Geometry: final body of the model. Coordinates: model frame, mm. A direction names the side the tool comes from. Coordinates: 2 decimals unless noted, no trailing zeros. Write each loop counter-clockwise with the first axis right and the second up, starting at its lowest first coordinate (ties: lowest second). Pieces come first, ordered by that corner, then holes. Notation, with made-up numbers: (77.5, -0.5) -> (130.5, -0.5) arc R26 cw to (130.5, 35.5) -> close; hole circle Ø10 at (54.5, -32). An arc over 180 degrees is marked (long way). One line per item, written item: value.
```python
from build123d import *

# Parameters (mm, degrees)
F0_R     = 26
F0_R_2   = 7
F1_DEPTH = 3
F2_DEPTH = 15
F3_SIZE2 = 1.819851
F3_SIZE  = 5
F4_SIZE2 = 1.819851
F4_SIZE  = 5


with BuildPart() as f1:
    # F0 (on Top) → F1 (new body)
    with BuildSketch(Plane.XY):
        Circle(F0_R)
        with BuildLine():
            ThreePointArc((3, 22.803509), (17.291616, 15.165751), (23, 0))
            ThreePointArc((23, 0), (22.557855, -4.488117), (21.248418, -8.803678))
            ThreePointArc((21.248418, -8.803678), (19.918584, -11.5), (18.248418, -13.99983))
            ThreePointArc((18.248418, -13.99983), (0, -23), (-18.248418, -13.99983))
            ThreePointArc((-18.248418, -13.99983), (-19.918584, -11.5), (-21.248418, -8.803678))
            ThreePointArc((-21.248418, -8.803678), (-19.918584, 11.5), (-3, 22.803509))
            ThreePointArc((-3, 22.803509), (0, 23), (3, 22.803509))
        make_face(mode=Mode.SUBTRACT)
        with BuildLine():
            Line((-9.761356, -2.17162), (-21.248418, -8.803678))
            ThreePointArc((-21.248418, -8.803678), (-19.918584, -11.5), (-18.248418, -13.99983))
            Line((-18.248418, -13.99983), (-6.761356, -7.367772))
            ThreePointArc((-6.761356, -7.367772), (-8.660254, -5), (-9.761356, -2.17162))
        make_face()
        with BuildLine():
            ThreePointArc((10, 0), (8.062258, 5.91608), (3, 9.539392))
            ThreePointArc((3, 9.539392), (0, 10), (-3, 9.539392))
            ThreePointArc((-3, 9.539392), (-8.660254, 5), (-9.761356, -2.17162))
            ThreePointArc((-9.761356, -2.17162), (-8.660254, -5), (-6.761356, -7.367772))
            ThreePointArc((-6.761356, -7.367772), (0, -10), (6.761356, -7.367772))
            ThreePointArc((6.761356, -7.367772), (8.660254, -5), (9.761356, -2.17162))
            ThreePointArc((9.761356, -2.17162), (9.94016, -1.092347), (10, 0))
        make_face()
        Circle(F0_R_2, mode=Mode.SUBTRACT)
        with BuildLine():
            Line((3, 9.539392), (3, 22.803509))
            ThreePointArc((3, 22.803509), (0, 23), (-3, 22.803509))
            Line((-3, 22.803509), (-3, 9.539392))
            ThreePointArc((-3, 9.539392), (0, 10), (3, 9.539392))
        make_face()
        with BuildLine():
            ThreePointArc((18.248418, -13.99983), (19.918584, -11.5), (21.248418, -8.803678))
            Line((21.248418, -8.803678), (9.761356, -2.17162))
            ThreePointArc((9.761356, -2.17162), (8.660254, -5), (6.761356, -7.367772))
            Line((6.761356, -7.367772), (18.248418, -13.99983))
        make_face()
    extrude(amount=F1_DEPTH)

    # F0 (on Top) → F2 (join)
    with BuildSketch(Plane.XY):
        Circle(F0_R)
        with BuildLine():
            ThreePointArc((3, 22.803509), (17.291616, 15.165751), (23, 0))
            ThreePointArc((23, 0), (22.557855, -4.488117), (21.248418, -8.803678))
            ThreePointArc((21.248418, -8.803678), (19.918584, -11.5), (18.248418, -13.99983))
            ThreePointArc((18.248418, -13.99983), (0, -23), (-18.248418, -13.99983))
            ThreePointArc((-18.248418, -13.99983), (-19.918584, -11.5), (-21.248418, -8.803678))
            ThreePointArc((-21.248418, -8.803678), (-19.918584, 11.5), (-3, 22.803509))
            ThreePointArc((-3, 22.803509), (0, 23), (3, 22.803509))
        make_face(mode=Mode.SUBTRACT)
        with BuildLine():
            ThreePointArc((10, 0), (8.062258, 5.91608), (3, 9.539392))
            ThreePointArc((3, 9.539392), (0, 10), (-3, 9.539392))
            ThreePointArc((-3, 9.539392), (-8.660254, 5), (-9.761356, -2.17162))
            ThreePointArc((-9.761356, -2.17162), (-8.660254, -5), (-6.761356, -7.367772))
            ThreePointArc((-6.761356, -7.367772), (0, -10), (6.761356, -7.367772))
            ThreePointArc((6.761356, -7.367772), (8.660254, -5), (9.761356, -2.17162))
            ThreePointArc((9.761356, -2.17162), (9.94016, -1.092347), (10, 0))
        make_face()
        Circle(F0_R_2, mode=Mode.SUBTRACT)
    extrude(amount=-F2_DEPTH)

    # F3
    f3_edges = [f1.edges().sort_by_distance(p)[0] for p in [
        (-26, 0, -15),
    ]]
    chamfer(f3_edges, length=F3_SIZE, length2=F3_SIZE2)

    # F4
    f4_edges = [f1.edges().sort_by_distance(p)[0] for p in [
        (-7, 0, -15),
    ]]
    chamfer(f4_edges, length=F4_SIZE, length2=F4_SIZE2)


solid = f1.part
```
(1) Reachability of faces 3 (the flat face through (3, 16, 1)), 4 (the flat face through (0, 16, 0)), 5 (the flat face through (0, -9, -15)) from +Z, -Z, +X, -X, +Y, -Y: full face, straight path, thin tool, end or side. Return the list, or none.
Responses:
face 3: +Z, -Z
face 4: -Z
face 5: -Z, +X, -X, +Y, -Y
(2) Pull-direction query (Y, two-part tool) for faces 1 (the flat face through (0, -8, 3)), 2 (the flat face through (-12.585, -10.73, 1.479)); classes: released by +Y, released by -Y, zero draft, split by the parting line, or undercut.
Responses:
face 1: zero draft
face 2: undercut
(3) Section D-D (y = 5). State how many separate pieces and enclosed holes the cut face has, then the cut area to 3 significant figures.
Responses:
separate pieces: 4
enclosed holes: 0
area: 224 mm2
(4) Line query: line 1 (Y direction, x = -9, z = -3); line 2 (Y direction, x = 5, z = -2); line 3 (Y direction, x = 3.5, z = -10.75). Output: solid intervals per line, ascending. Write a range as [from, to].
Responses:
line 1: y = [-24.39, -21.17], [-4.36, 4.36], [21.17, 24.39]
line 2: y = [-25.51, -22.45], [-8.66, -4.9], [4.9, 8.66], [22.45, 25.51]
line 3: y = [-25.49, -22.73], [-9.37, -6.38], [6.38, 9.37], [22.73, 25.49]
(5) Section C-C (z = -12.5). Return the cut outline in (x, y).
Responses:
outline: circle Ø50.18 at (0, 0); (-9.76, -2.17) arc R10 ccw to (-6.76, -7.37) arc R10 ccw to (6.76, -7.37) arc R10 ccw to (9.76, -2.17) arc R10 ccw to (10, 0) arc R10 ccw to (3, 9.54) arc R10 ccw to start; hole (-21.25, -8.8) arc R23 ccw to (-18.25, -14) arc R23 ccw to (18.25, -14) arc R23 ccw to (21.25, -8.8) arc R23 ccw to (23, 0) arc R23 ccw to (3, 22.8) arc R23 ccw to (-3, 22.8) arc R23 ccw to start; hole circle Ø15.82 at (0, 0)
(6) Section B-B (x = 0). Return the cut outline in (y, z).
Responses:
outline: (-26, -10) -> (-24.18, -15) -> (-23, -15) -> (-23, 3) -> (-26, 3) -> close; (-10, -15) -> (-8.82, -15) -> (-7, -10) -> (-7, 3) -> (-10, 3) -> close; (7, -10) -> (8.82, -15) -> (10, -15) -> (10, 0) -> (23, 0) -> (23, -15) -> (24.18, -15) -> (26, -10) -> (26, 3) -> (7, 3) -> close
(7) Section A-A (z = -6.75). Return the cut outline in (x, y), then the cut area to 3 significant figures.
Responses:
outline: circle Ø52 at (0, 0); (-9.76, -2.17) arc R10 ccw to (-6.76, -7.37) arc R10 ccw to (6.76, -7.37) arc R10 ccw to (9.76, -2.17) arc R10 ccw to (10, 0) arc R10 ccw to (3, 9.54) arc R10 ccw to start; hole (-21.25, -8.8) arc R23 ccw to (-18.25, -14) arc R23 ccw to (18.25, -14) arc R23 ccw to (21.25, -8.8) arc R23 ccw to (23, 0) arc R23 ccw to (3, 22.8) arc R23 ccw to (-3, 22.8) arc R23 ccw to start; hole circle Ø14 at (0, 0)
area: 622 mm2
(8) First-contact query: pin 1 (3 mm diameter, centred on x = 9.5, z = -5, fed in from -Y); pin 2 (4 mm diameter, centred on x = -11.5, z = -3, fed in from -Y); pin 3 (1.5 mm diameter, centred on y = 16.5, z = 2, fed in from +X). Flat tips, straight axial feed; report the tip coordinate or a pass-through.
Responses:
pin 1: stops at y = -24.74
pin 2: stops at y = -24.2
pin 3: stops at x = 20.69
